Answer from the drawing. Dimensions are ordinates in mm from the lowest x, y and z of the part. A direction names the side the tool comes from. Coordinates: 2 decimals unless noted, no trailing zeros. Loops run counter-clockwise (first coordinate to the right, second up) from the corner with the lowest first, then second, coordinate; pieces in that order, holes last. Notation, with made-up numbers: M 56.25,12 L 112.25,12 A17 ccw 112.25,38 Z; hole C -35.75,-1.75 d1. An arc over 180 degrees is marked long. Answer as CSV lines item,"result". Start each with the question number.
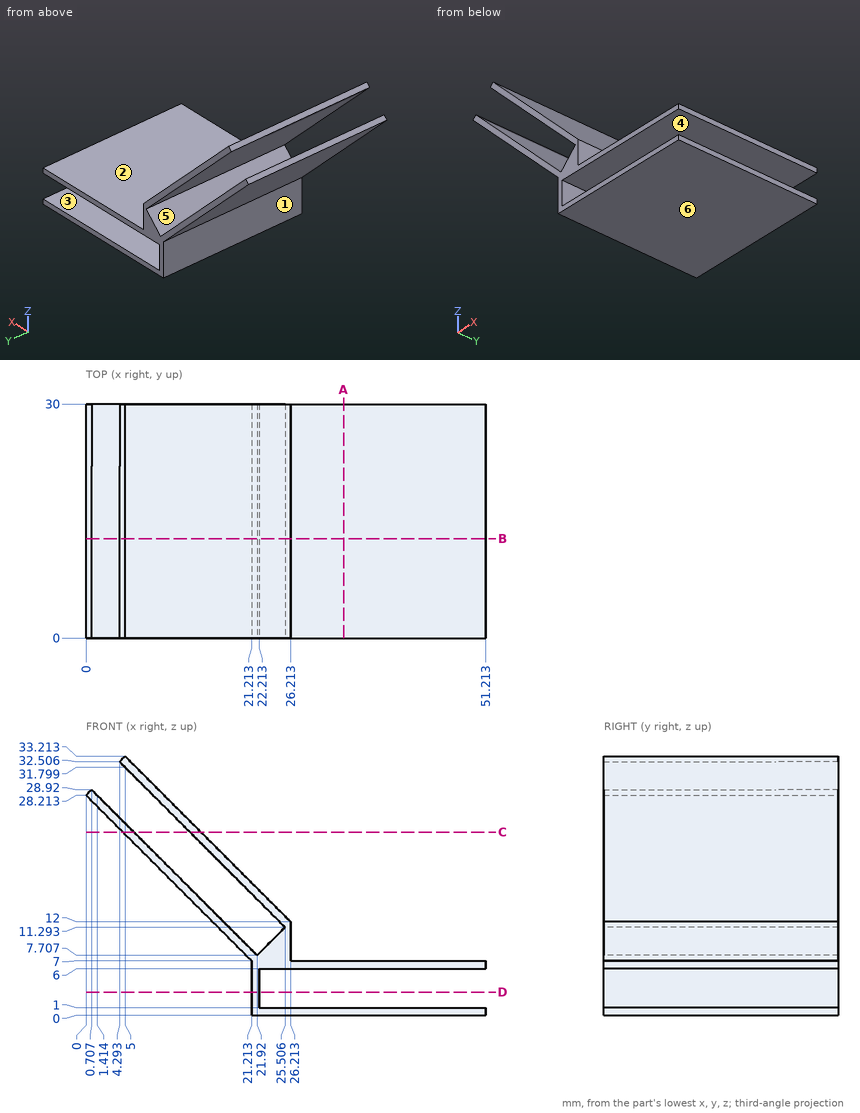
Item 1: Section A-A on x = 33 is taken. Determine the outline of the cut face in (y, z).
Item 2: For a pull along Z with two mould halves and no side action, classify the marked faces 1, 2 and 3 as pulls with the +Z half, pulls with the -Z half, needs draft (parallel to the pull), parting line crosses it, or undercut.
Item 3: Each of these flat-tipped pins is pushed along its axis until it touches: P1, Ø2.5, axis at y = 13.5, z = 4.5, coming from the +X side; P2, Ø1.5, axis at x = 18.5, y = 3, coming from the -Z side; P3, Ø12.5, axis at x = 38, y = 12, coming from the +Z side. Where does it stop, or does it pass through?
Item 4: Section C-C on z = 23.5 is taken. Determine the outline of the cut face in (x, y).
Item 5: For the marked faces 4, 5 and 6, determine the directions among +Z, -Z, +X, -X, +Y, -Y from which every point of the face is accessible in a straight line to the end or side of a thin tool.
Item 6: Section B-B on y = 12.75 is taken. Determine the outline of the cut face in (x, z).
Item 7: Section D-D on z = 3 is taken. Determine the outline of the cut face in (x, y), then the cut area to 3 significant figures.
Item 8: Consider line 1 (Z direction, x = 35.5, y = 24); line 2 (Z direction, x = 25, y = 21.75) (1 decimal); line 3 (X direction, y = 21.5, z = 13) (1 decimal). Determine where each line is inside the solid, lowest interval first.
Results are:
1,outline,"M 0,0 L 30,0 L 30,1 L 0,1 Z; M 0,6 L 30,6 L 30,7 L 0,7 Z"
2,face 1,"needs draft"
2,face 2,"pulls with the +Z half"
2,face 3,"undercut"
3,P1,"x = 22.21"
3,P2,"z = 8.96"
3,P3,"z = 7"
4,outline,"M 4.71,0 L 6.13,0 L 6.13,30 L 4.71,30 Z; M 13.3,0 L 14.71,0 L 14.71,30 L 13.3,30 Z"
5,face 4,"+X, +Y, -Y"
5,face 5,"+Y, -Y"
5,face 6,"-Z, +X, -X, +Y, -Y"
6,outline,"M 0,28.21 L 21.21,7 L 21.21,0 L 51.21,0 L 51.21,1 L 22.21,1 L 22.21,6 L 51.21,6 L 51.21,7 L 26.21,7 L 26.21,12 L 5,33.21 L 4.29,32.51 L 25.51,11.29 L 21.92,7.71 L 0.71,28.92 Z"
7,outline,"M 21.21,0 L 22.21,0 L 22.21,30 L 21.21,30 Z"
7,area,"30.0 mm²"
8,line 1,"0 to 1, 6 to 7"
8,line 2,"0 to 1, 6 to 10.8, 11.8 to 13.2"
8,line 3,"15.2 to 16.6, 23.8 to 25.2"
